```python
from build123d import *

# Parameters (mm, degrees)
SKETCH1_W                   = 42.3
SKETCH1_H                   = 42.3
BOSS_EXTRUDE1_DEPTH         = 48
SKETCH2_R                   = 11
BOSS_EXTRUDE2_DEPTH         = 2
SKETCH3_R                   = 2.5
BOSS_EXTRUDE3_DEPTH         = 22
CHAMFER1_SIZE               = 0.5
CHAMFER2_SIZE               = 4
M3_TAPPED_HOLE1_D           = 2.5
M3_TAPPED_HOLE1_DEPTH       = 4.5
M3_TAPPED_HOLE1_CSINK_D     = 3.05
M3_TAPPED_HOLE1_CSINK_ANGLE = 90
M3_TAPPED_HOLE1_TIP         = 0.751075774
SKETCH5_R                   = 2.5
BOSS_EXTRUDE4_DEPTH         = 10


with BuildPart() as part:
    # Sketch1 → Boss-Extrude1 (new body)
    with BuildSketch(Plane.XY):
        Rectangle(SKETCH1_W, SKETCH1_H)
    extrude(amount=BOSS_EXTRUDE1_DEPTH)

    # Sketch2 → Boss-Extrude2 (add)
    with BuildSketch(Plane.XY.offset(48)):
        Circle(SKETCH2_R)
    extrude(amount=BOSS_EXTRUDE2_DEPTH)

    # Sketch3 → Boss-Extrude3 (add)
    with BuildSketch(Plane.XY.offset(50)):
        Circle(SKETCH3_R)
    extrude(amount=BOSS_EXTRUDE3_DEPTH)

    # Chamfer1
    chamfer1_edges = [part.edges().sort_by_distance(p)[0] for p in [
        (-2.5, 0, 72),
    ]]
    chamfer(chamfer1_edges, length=CHAMFER1_SIZE)

    # Chamfer2
    chamfer2_edges = [part.edges().sort_by_distance(p)[0] for p in [
        (-21.15, 21.15, 24),
        (21.15, 21.15, 24),
        (21.15, -21.15, 24),
        (-21.15, -21.15, 24),
    ]]
    chamfer(chamfer2_edges, length=CHAMFER2_SIZE)

    # M3 Tapped Hole1
    with Locations(Plane(origin=(-15.5, 15.5, 48), x_dir=(1, 0, 0), z_dir=(0, 0, 1))):
        with Locations((0, 0), (31, 0), (31, -31), (0, -31)):
            CounterSinkHole(M3_TAPPED_HOLE1_D / 2, M3_TAPPED_HOLE1_CSINK_D / 2, depth=M3_TAPPED_HOLE1_DEPTH, counter_sink_angle=M3_TAPPED_HOLE1_CSINK_ANGLE)
            with Locations((0, 0, -(M3_TAPPED_HOLE1_DEPTH + M3_TAPPED_HOLE1_TIP / 2))):  # 118° drill point
                Cone(0, M3_TAPPED_HOLE1_D / 2, M3_TAPPED_HOLE1_TIP, mode=Mode.SUBTRACT)

    # Sketch5 → Boss-Extrude4 (add)
    with BuildSketch(Plane.XZ.offset(21.15)):
        with Locations(Location((0, 8, 0), (0, 0, 90))):
            Circle(SKETCH5_R)
    extrude(amount=BOSS_EXTRUDE4_DEPTH)


solid = part.part
```
For this review, take the finished solid that the model builds, in its own axes (mm). A direction names the side the tool comes from. Coordinates: 2 decimals unless noted, no trailing zeros. Write each loop counter-clockwise with the first axis right and the second up, starting at its lowest first coordinate (ties: lowest second). Pieces come first, ordered by that corner, then holes. Notation, with made-up numbers: (39, -5) - (56, -5) arc R26 ccw to (56, 15) - close; hole circle Ø5 at (74.5, 45.5). An arc over 180 degrees is marked (long way). Put each result on its own line as item: value.
1. Add section C-C, the plane x = -4. Give the boundary of the cut face in (y, z), then the cut area to 3 significant figures.
Values found:
outline: (-21.15, 0) - (21.15, 0) - (21.15, 48) - (10.25, 48) - (10.25, 50) - (-10.25, 50) - (-10.25, 48) - (-21.15, 48) - close
area: 2,070 mm²
2. Machinability: for faces 5 (the flat face through (0, 21.15, 24)), 6 (the flat face through (-10, -9, 48)), which of the approach directions +Z, -Z, +X, -X, +Y, -Y give a long, thin tool a straight path to every point of the face, cutting with its end or side? Answer none if there is none.
Values found:
face 5: +Z, -Z, +X, -X, +Y
face 6: +Z
3. Add section A-A, the plane z = 19. Give the boundary of the cut face in (x, y).
Values found:
outline: (-21.15, -17.15) - (-17.15, -21.15) - (17.15, -21.15) - (21.15, -17.15) - (21.15, 17.15) - (17.15, 21.15) - (-17.15, 21.15) - (-21.15, 17.15) - close
4. Add section D-D, the plane z = 8. Give the boundary of the cut face in (x, y), then the cut area to 3 significant figures.
Values found:
outline: (-21.15, -17.15) - (-17.15, -21.15) - (-2.5, -21.15) - (-2.5, -31.15) - (2.5, -31.15) - (2.5, -21.15) - (17.15, -21.15) - (21.15, -17.15) - (21.15, 17.15) - (17.15, 21.15) - (-17.15, 21.15) - (-21.15, 17.15) - close
area: 1,810 mm²
5. Mouldability with a two-part tool opening along X and no side actions: class faces 1 (the cylindrical face through (-0.751, -26.08, 10.385)), 2 (the cylindrical face through (-15.34, -14.26, 45.58)), 3 (the flat face through (19.2, -19.1, 23.7)), 4 (the flat face through (0, -21.15, 24)) as released by +X, released by -X, zero draft, split by the parting line, or undercut.
Values found:
face 1: split by the parting line
face 2: undercut
face 3: released by +X
face 4: zero draft
6. Wall thickness on probe 1 along Y at (x, z) = (15.5, 44.95); probe 2 along X at (y, z) = (-15, 44): over which ranges is each line inside the solid? List them lowest first.
Values found:
probe 1: -21.15 to -16.75, -14.25 to 14.25, 16.75 to 21.15
probe 2: -21.15 to -16.65, -14.35 to 14.35, 16.65 to 21.15
7. For pin 1 (1.5 mm diameter, centred on x = -15.5, y = -15.5, fed in from +Z); pin 2 (3 mm diameter, centred on x = 15.5, y = -15.5, fed in from +Z) (3 decimals); pin 3 (3 mm diameter, centred on x = -8, z = 48.5, fed in from -Y), all flat-tipped, find the tip position at first contact; note any pin that passes through.
Values found:
pin 1: z = 43.2
pin 2: z = 47.975
pin 3: y = -21.15
8. Add section B-B, the plane y = 0. Give the boundary of the cut face in (x, z).
Values found:
outline: (-21.15, 0) - (21.15, 0) - (21.15, 48) - (11, 48) - (11, 50) - (2.5, 50) - (2.5, 71.5) - (2, 72) - (-2, 72) - (-2.5, 71.5) - (-2.5, 50) - (-11, 50) - (-11, 48) - (-21.15, 48) - close
